Geometry check sheet. Reference: the model listing, model coordinates, mm. Face numbers are marked on the shaded views. A direction names the side the tool comes from. Give positions to 0.01 mm unless a question says otherwise; leave off trailing zeros. Write each loop counter-clockwise with the first axis right and the second up, starting at its lowest first coordinate (ties: lowest second). Pieces come first, ordered by that corner, then holes. Notation, with made-up numbers: (-0.5, 76.5) -> (52.5, 76.5) arc R30 cw to (52.5, 114.5) -> close; hole circle Ø4 at (-25.75, 23.25). An arc over 180 degrees is marked (long way). Write item = value, one per line. Start each with the question number.
1. Set-up check for the marked faces 4, 5, 6 and 7: record each of +Z, -Z, +X, -X, +Y, -Y from which the full face is reachable in a straight line by a thin tool's end or side.
2. Thickness scan on line 1 along Y through (x, z) = (0, 36); line 2 along Y through (x, z) = (6.5, 37); line 3 along X through (y, z) = (3, 48.5). Record the ranges inside material, lowest first.
3. Cross-section at A-A, the plane z = 28.5. Record the cut outline in (x, y).
4. Cross-section at C-C, the plane y = 22.5. State how many separate pieces and enclosed holes the cut face has, plus the area to 3 significant figures.
5. Cross-section at D-D, the plane x = -6. Record the cut outline in (y, z).
6. Mould release check, pull along X, two halves, no side actions. Record for the marked faces 1, 2 and 3: pulls with the +X half, pulls with the -X half, needs draft (parallel to the pull), parting line crosses it, or undercut.
7. Cross-section at B-B, the plane z = 46. Record the cut outline in (x, y), plus the area to 3 significant figures.
8. Depth check by flat-ended pin: P1, Ø5, axis at y = 6.5, z = 22.5, coming from the -X side; P2, Ø6, axis at x = -8, y = 23.5, coming from the -Z side; P3, Ø3, axis at y = 3, z = 14.5, coming from the +X side. Enter the tip coordinate at first touch or a pass-through.
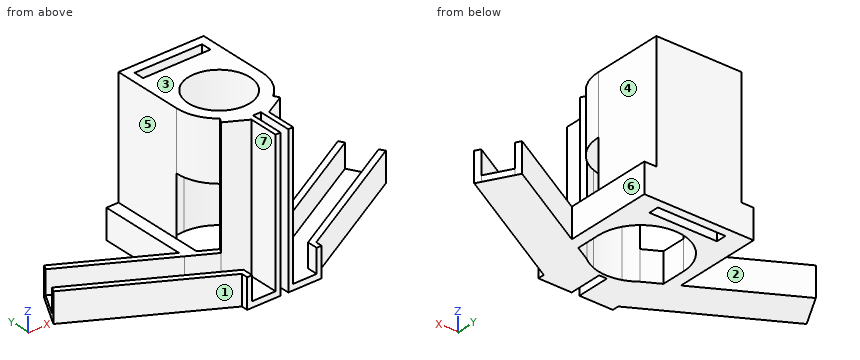
```python
from build123d import *

# Parameters (mm, degrees)
F1_DEPTH = 10
F2_DEPTH = 2
F0_R     = 10.5
F3_DEPTH = 50
F4_DEPTH = 30
F0_W     = 23
F0_H     = 3.5
F5_DEPTH = 50


with BuildPart() as f1:
    # F0 (on Top) → F1 (new body)
    with BuildSketch(Plane.XY):
        Polygon((-12.6842105263, 0), (-11, 0), (-11, 3.5898238607), (-55.6379765465, 28.5605340733), (-56.6143926616, 26.8150795278), (-12.6842105263, 2.2403130945), align=None)
    extrude(amount=F1_DEPTH)



with BuildPart() as f1b:
    # F0 (on Top) → F1, piece 2 (new body)
    with BuildSketch(Plane.XY):
        Polygon((-51, 36.8514431642), (-18.596614075, 18.7248249248), (-18.596614075, 21.0164915914), (-50.0235838849, 38.5968977096), align=None)
        Polygon((-18.596614075, 21.0164915914), (-18.596614075, 18.7248249248), (-14.5, 18.7248249248), align=None)
        Polygon((-18.596614075, 21.0164915914), (-14.5, 18.7248249248), (-14.5, 27), (-14.5, 41.5), (-14.5, 51), (-18.596614075, 51), align=None)
        Polygon((-18.596614075, 18.7248249248), (-10.0476759502, 13.9425056295), (-9.0712598352, 15.687960175), (-14.5, 18.7248249248), align=None)
    extrude(amount=F1_DEPTH)


with BuildPart() as f1c:
    # F0 (on Top) → F1, piece 3 (new body)
    with BuildSketch(Plane.XY):
        Polygon((18.596614075, 21.0164915914), (14.5, 18.7248249248), (18.596614075, 18.7248249248), align=None)
        Polygon((18.596614075, 21.0164915914), (18.596614075, 18.7248249248), (51, 36.8514431642), (50.0235838849, 38.5968977096), align=None)
        Polygon((14.5, 51), (14.5, 41.5), (14.5, 27), (14.5, 18.7248249248), (18.596614075, 21.0164915914), (18.596614075, 51), align=None)
        Polygon((14.5, 18.7248249248), (9.0712598352, 15.687960175), (10.0476759502, 13.9425056295), (18.596614075, 18.7248249248), align=None)
    extrude(amount=F1_DEPTH)



with BuildPart() as f1d:
    # F0 (on Top) → F1, piece 4 (new body)
    with BuildSketch(Plane.XY):
        Polygon((55.6379765465, 28.5605340733), (11, 3.5898238607), (12.6842105263, 2.2403130945), (56.6143926616, 26.8150795278), align=None)
        Polygon((11, 3.5898238607), (11, 0), (12.6842105263, 0), (12.6842105263, 2.2403130945), align=None)
    extrude(amount=F1_DEPTH)


with BuildPart() as f1_1:
    add(f1.part)

    add(f1b.part)  # F2 merges F1b
    # F0 (on Top) → F2 (join)
    with BuildSketch(Plane.XY):
        Polygon((-11, 0), (-3, 0), (-3, 10), (-10.0476759502, 13.9425056295), (-18.596614075, 18.7248249248), (-51, 36.8514431642), (-55.6379765465, 28.5605340733), (-11, 3.5898238607), align=None)
    extrude(amount=F2_DEPTH)



with BuildPart() as f1c_1:
    add(f1c.part)

    add(f1d.part)  # F2#2 merges F1d
    # F0 (on Top) → F2, piece 2 (join)
    with BuildSketch(Plane.XY):
        Polygon((10.0476759502, 13.9425056295), (3, 10), (11, 3.5898238607), (55.6379765465, 28.5605340733), (51, 36.8514431642), (18.596614075, 18.7248249248), align=None)
        Polygon((3, 10), (3, 0), (11, 0), (11, 3.5898238607), align=None)
    extrude(amount=F2_DEPTH)


with BuildPart() as f1_2:
    add(f1_1.part)

    add(f1c_1.part)  # F3 merges F1c
    # F0 (on Top) → F3 (join)
    with BuildSketch(Plane.XY):
        with BuildLine():
            ThreePointArc((-14.5, 27), (-13.0725526889, 20.7263753543), (-9.0712598352, 15.687960175))
            Line((-9.0712598352, 15.687960175), (-4.8924551228, 13.3503156494))
            ThreePointArc((-4.8924551228, 13.3503156494), (0, 12.5), (4.8924551228, 13.3503156494))
            Line((4.8924551228, 13.3503156494), (9.0712598352, 15.687960175))
            ThreePointArc((9.0712598352, 15.687960175), (13.0725526889, 20.7263753543), (14.5, 27))
            ThreePointArc((14.5, 27), (10.2530483272, 37.2530483272), (0, 41.5))
            ThreePointArc((0, 41.5), (-10.2530483272, 37.2530483272), (-14.5, 27))
        make_face()
        with Locations((0, 27)):
            Circle(F0_R, mode=Mode.SUBTRACT)
        with BuildLine():
            Line((-4.8924551228, 13.3503156494), (-9.0712598352, 15.687960175))
            ThreePointArc((-9.0712598352, 15.687960175), (-7.0790168342, 14.3454545455), (-4.8924551228, 13.3503156494))
        make_face()
        with BuildLine():
            Line((9.0712598352, 15.687960175), (4.8924551228, 13.3503156494))
            ThreePointArc((4.8924551228, 13.3503156494), (7.0790168342, 14.3454545455), (9.0712598352, 15.687960175))
        make_face()
    extrude(amount=F3_DEPTH)

    # F0 (on Top) → F4 (cut)
    with BuildSketch(Plane.XY):
        with BuildLine():
            ThreePointArc((-14.5, 27), (-13.0725526889, 20.7263753543), (-9.0712598352, 15.687960175))
            Line((-9.0712598352, 15.687960175), (-4.8924551228, 13.3503156494))
            ThreePointArc((-4.8924551228, 13.3503156494), (0, 12.5), (4.8924551228, 13.3503156494))
            Line((4.8924551228, 13.3503156494), (9.0712598352, 15.687960175))
            ThreePointArc((9.0712598352, 15.687960175), (13.0725526889, 20.7263753543), (14.5, 27))
            ThreePointArc((14.5, 27), (10.2530483272, 37.2530483272), (0, 41.5))
            ThreePointArc((0, 41.5), (-10.2530483272, 37.2530483272), (-14.5, 27))
        make_face()
        with Locations((0, 27)):
            Circle(F0_R, mode=Mode.SUBTRACT)
        with BuildLine():
            Line((-4.8924551228, 13.3503156494), (-9.0712598352, 15.687960175))
            ThreePointArc((-9.0712598352, 15.687960175), (-7.0790168342, 14.3454545455), (-4.8924551228, 13.3503156494))
        make_face()
        with BuildLine():
            Line((9.0712598352, 15.687960175), (4.8924551228, 13.3503156494))
            ThreePointArc((4.8924551228, 13.3503156494), (7.0790168342, 14.3454545455), (9.0712598352, 15.687960175))
        make_face()
    extrude(amount=F4_DEPTH, mode=Mode.SUBTRACT)

    # F0 (on Top) → F5 (join)
    with BuildSketch(Plane.XY):
        with BuildLine():
            Line((-14.5, 41.5), (-14.5, 27))
            ThreePointArc((-14.5, 27), (-10.2530483272, 37.2530483272), (0, 41.5))
            Line((0, 41.5), (-14.5, 41.5))
        make_face()
        with BuildLine():
            Line((14.5, 41.5), (0, 41.5))
            ThreePointArc((0, 41.5), (10.2530483272, 37.2530483272), (14.5, 27))
            Line((14.5, 27), (14.5, 41.5))
        make_face()
        with BuildLine():
            Line((-4.8924551228, 13.3503156494), (-1.3157894737, 11.3495107662))
            Line((-1.3157894737, 11.3495107662), (1.3157894737, 11.3495107662))
            Line((1.3157894737, 11.3495107662), (4.8924551228, 13.3503156494))
            ThreePointArc((4.8924551228, 13.3503156494), (0, 12.5), (-4.8924551228, 13.3503156494))
        make_face()
        Polygon((-14.5, 41.5), (0, 41.5), (14.5, 41.5), (14.5, 51), (-14.5, 51), align=None)
        with Locations((0, 46.25)):
            Rectangle(F0_W, F0_H, mode=Mode.SUBTRACT)
        with BuildLine():
            Line((1.3157894737, 11.3495107662), (1.3157894737, 0))
            Line((1.3157894737, 0), (3, 0))
            Line((3, 0), (3, 10))
            Line((3, 10), (10.0476759502, 13.9425056295))
            Line((10.0476759502, 13.9425056295), (9.0712598352, 15.687960175))
            ThreePointArc((9.0712598352, 15.687960175), (7.0790168342, 14.3454545455), (4.8924551228, 13.3503156494))
            Line((4.8924551228, 13.3503156494), (1.3157894737, 11.3495107662))
        make_face()
        with BuildLine():
            Line((-3, 10), (-3, 0))
            Line((-3, 0), (-1.3157894737, 0))
            Line((-1.3157894737, 0), (-1.3157894737, 11.3495107662))
            Line((-1.3157894737, 11.3495107662), (-4.8924551228, 13.3503156494))
            ThreePointArc((-4.8924551228, 13.3503156494), (-7.0790168342, 14.3454545455), (-9.0712598352, 15.687960175))
            Line((-9.0712598352, 15.687960175), (-10.0476759502, 13.9425056295))
            Line((-10.0476759502, 13.9425056295), (-3, 10))
        make_face()
    extrude(amount=F5_DEPTH)


solid = f1_2.part
```
Answers:
q1.face_4 = +Z, +X, +Y, -Y
q1.face_5 = +Z, -X, +Y, -Y
q1.face_6 = +Z, -Z, +Y
q1.face_7 = +Z, -Y
q2.line_1 = 11.35 to 16.5, 37.5 to 44.5, 48 to 51
q2.line_2 = 11.96 to 18.75, 35.25 to 44.5, 48 to 51
q2.line_3 = -3 to -1.32, 1.32 to 3
q3.outline = (-14.5, 27) arc R14.5 cw to (14.5, 27) -> (14.5, 51) -> (-14.5, 51) -> close; (-10.05, 13.94) -> (-3, 10) -> (-3, 0) -> (-1.32, 0) -> (-1.32, 11.35) -> (1.32, 11.35) -> (1.32, 0) -> (3, 0) -> (3, 10) -> (10.05, 13.94) -> (9.07, 15.69) arc R14.5 cw to (-9.07, 15.69) -> close; hole (-11.5, 44.5) -> (11.5, 44.5) -> (11.5, 48) -> (-11.5, 48) -> close
q4.separate_pieces = 6
q4.enclosed_holes = 0
q4.area = 496 mm^2
q5.outline = (0, 0) -> (13.8, 0) -> (13.8, 30) -> (18.38, 30) -> (18.38, 50) -> (11.68, 50) -> (11.68, 2) -> (0, 2) -> close; (35.62, 30) -> (40.2, 30) -> (40.2, 0) -> (44.5, 0) -> (44.5, 50) -> (35.62, 50) -> close; (48, 0) -> (51, 0) -> (51, 50) -> (48, 50) -> close
q6.face_1 = pulls with the -X half
q6.face_2 = undercut
q6.face_3 = needs draft
q7.outline = (-14.5, 27) arc R14.5 ccw to (-9.07, 15.69) -> (-10.05, 13.94) -> (-3, 10) -> (-3, 0) -> (-1.32, 0) -> (-1.32, 11.35) -> (1.32, 11.35) -> (1.32, 0) -> (3, 0) -> (3, 10) -> (10.05, 13.94) -> (9.07, 15.69) arc R14.5 ccw to (14.5, 27) -> (14.5, 51) -> (-14.5, 51) -> close; hole (-11.5, 44.5) -> (11.5, 44.5) -> (11.5, 48) -> (-11.5, 48) -> close; hole circle Ø21 at (0, 27)
q7.area = 675 mm^2
q8.P1 = -3
q8.P2 = 30
q8.P3 = 3
